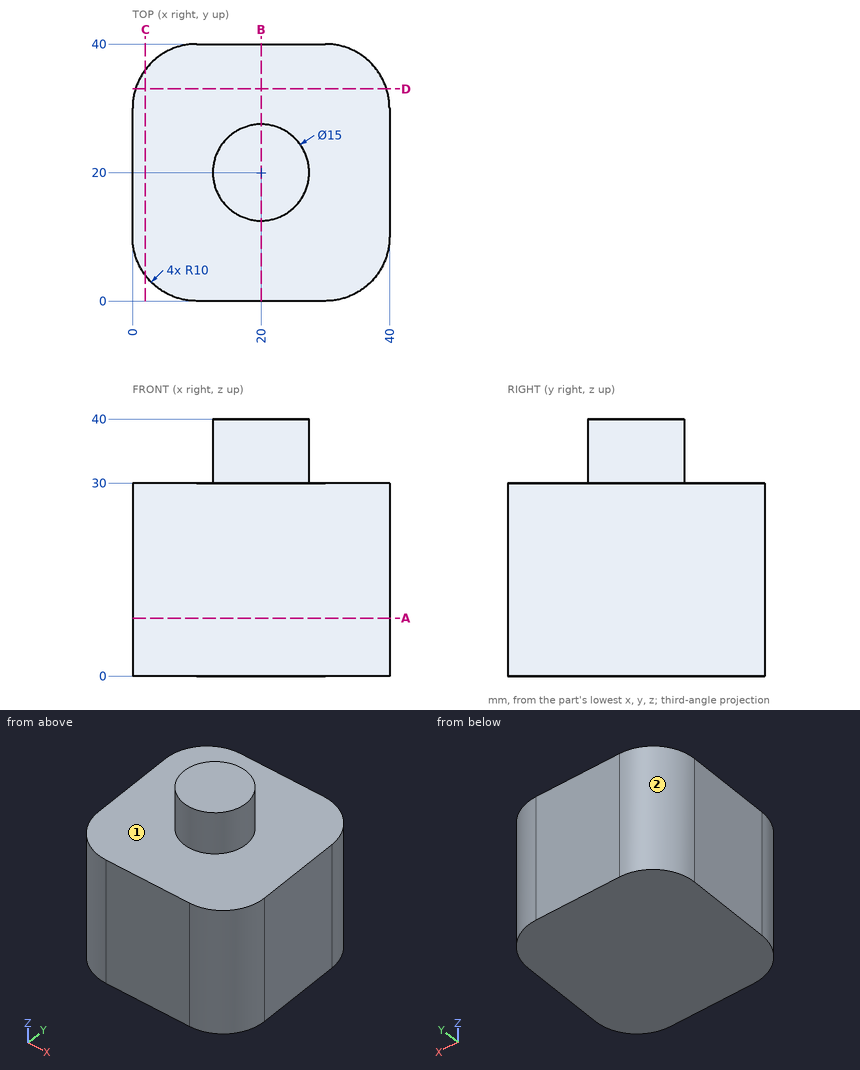
Here's the drawing with two shaded views (mm, measured from the low corner). I have some questions. A direction names the side the tool comes from. Give positions to 0.01 mm unless a question says otherwise; leave off trailing zeros. Loops run counter-clockwise (first coordinate to the right, second up) from the corner with the lowest first, then second, coordinate; pieces in that order, holes last. Notation, with made-up numbers: (-18.75, -28.75) -> (4.25, -28.75) arc R29 cw to (4.25, 9.25) -> close; hole circle Ø8 at (4.25, -15.5). An arc over 180 degrees is marked (long way). One line per item, written item: value.
Q1. On a 3-axis mill with a long thin cutter (end or side, diameter ignored), from which of +Z, -Z, +X, -X, +Y, -Y can I reach the whole of each face in a straight line? I mean the marked faces 1 and 2. Say none if no direction works.
Answers follow:
face 1: +Z
face 2: +Z, -Z, -X, +Y
Q2. Suppose I cut it at A-A on z = 9. Please give me the cut outline in (x, y).
Answers follow:
outline: (0, 10) arc R10 ccw to (10, 0) -> (30, 0) arc R10 ccw to (40, 10) -> (40, 30) arc R10 ccw to (30, 40) -> (10, 40) arc R10 ccw to (0, 30) -> close
Q3. Suppose I cut it at B-B on x = 20. Please give me the cut outline in (y, z), then the cut area to 3 significant figures.
Answers follow:
outline: (0, 0) -> (40, 0) -> (40, 30) -> (27.5, 30) -> (27.5, 40) -> (12.5, 40) -> (12.5, 30) -> (0, 30) -> close
area: 1,350 mm^2
Q4. Suppose I cut it at C-C on x = 2. Please give me the cut outline in (y, z).
Answers follow:
outline: (4, 0) -> (36, 0) -> (36, 30) -> (4, 30) -> close
Q5. I'm going to push flat-ended pins straight in: pin 1 Ø2 at (x, z) = (27.5, 15) entering from -Y; pin 2 Ø1.5 at (x, y) = (28, 23.5) entering from +Z; pin 3 Ø1.5 at (y, z) = (7.5, 12) entering from +X. Where does each tip first touch, or does it pass through?
Answers follow:
pin 1: y = 0
pin 2: z = 30
pin 3: x = 39.85
Q6. Suppose I cut it at D-D on y = 33. Please give me the cut outline in (x, z), then the cut area to 3 significant figures.
Answers follow:
outline: (0.46, 0) -> (39.54, 0) -> (39.54, 30) -> (0.46, 30) -> close
area: 1,170 mm^2
Q7. If I drill on line 1 along Z through (x, y) = (6, 2.5); line 2 along Y through (x, z) = (8, 19.5); line 3 along Y through (x, z) = (38, 8.5), over which ranges is the centre line in solid material (lowest first)?
Answers follow:
line 1: 0 to 30
line 2: 0.2 to 39.8
line 3: 4 to 36
